```python
from build123d import *

# Parameters (mm, degrees)
CHAMFER_1_SIZE = 0.4
CHAMFER_2_SIZE = 0.4
FILLET_1_R     = 0.5


with BuildPart() as part:
    # Эскиз1 → Повернуть1 (revolve)
    with BuildSketch(Plane(origin=(0, 0, 0), x_dir=(1, 0, 0), z_dir=(0, 1, 0))):
        Polygon((0, 31), (-1.5, 31), (-1.5, 27.3), (-1.1, 27.3), (-1.1, 26), (-2, 26), (-2, -26), (-1.1, -26), (-1.1, -27.3), (-1.5, -27.3), (-1.5, -31), (0, -31), align=None)
    revolve(axis=Axis((0, 0, -31), (0, 0, 1)))

    # Фаска1
    chamfer_1_edges = [part.edges().sort_by_distance(p)[0] for p in [
        (1.5, 0, -31),
        (1.5, 0, 31),
    ]]
    chamfer(chamfer_1_edges, length=CHAMFER_1_SIZE)

    # Фаска2
    chamfer_2_edges = [part.edges().sort_by_distance(p)[0] for p in [
        (1.5, 0, -27.3),
        (1.5, 0, 27.3),
    ]]
    chamfer(chamfer_2_edges, length=CHAMFER_2_SIZE - 0.0001)  # a hair under: the kernel refuses the full size

    # Скругление1
    fillet_1_edges = [part.edges().sort_by_distance(p)[0] for p in [
        (1.1, 0, -26),
        (1.1, 0, 26),
    ]]
    fillet(fillet_1_edges, radius=FILLET_1_R)


solid = part.part
```
Here's how the part is built. I have some questions about the finished solid (model axes, mm). A direction names the side the tool comes from. Give positions to 0.01 mm unless a question says otherwise; leave off trailing zeros. Write each loop counter-clockwise with the first axis right and the second up, starting at its lowest first coordinate (ties: lowest second). Pieces come first, ordered by that corner, then holes. Notation, with made-up numbers: M 64,-5.5 L 70,-5.5 A22 cw 70,14.5 Z; hole C -32,-31.75 d5. An arc over 180 degrees is marked long. Put each result on its own line as item: value. Start each with the question number.
Item 1: Thinking about a two-plate mould opening in Z: for faces 4 (the cylindrical face through (1.5, -0.07, -29.13)), 5 (the cylindrical face through (-1.05, -0.33, 26.91)), 6 (the flat face through (0, 0, 31)), which applies, +Z half, -Z half, draft (parallel to the pull), parting line (faces both ways), or undercut?
Item 2: I need wall thicknesses on L1, parallel to Z at x = 0.95, y = 0.9; L2, parallel to Y at x = 0.1, z = 0; L3, parallel to Z at x = -0.85, y = -1.1. Which ranges of each line are inside material? Lowest first, please. Write a range as from..to.
Item 3: If we section it at C-C, the plane z = 21: Write out the boundary of the cut face in (x, y).
Item 4: On a 3-axis mill with a long thin cutter (end or side, diameter ignored), from which of +Z, -Z, +X, -X, +Y, -Y can I reach the whole of each face in a straight line? I mean faces 1 (the cylindrical face through (-1.05, -0.33, -26.89)), 2 (the cylindrical face through (1.5, -0.07, 29.17)), 3 (the flat face through (0, 0, -31)). Say none if no direction works.
Values:
1. face 4: draft
1. face 5: undercut
1. face 6: +Z half
2. L1: -30.79..-27.51, -26.09..26.09, 27.51..30.79
2. L2: -2..2
2. L3: -30.71..-27.59, -26.05..26.05, 27.59..30.71
3. outline: C 0,0 d4
4. face 1: none
4. face 2: +Z
4. face 3: -Z, +X, -X, +Y, -Y
